Model file for the job. Use its own axes, mm. Round coordinates to 2 decimals unless told otherwise and drop trailing zeros. Loops run counter-clockwise (first coordinate to the right, second up) from the corner with the lowest first, then second, coordinate; pieces in that order, holes last. Notation, with made-up numbers: M 9,3.25 L 60,3.25 A15 ccw 60,20.25 Z; hole C -13.75,-22 d1. An arc over 180 degrees is marked long. Use a Markdown table: item, result. Add a question column.
Q1. Pin check, flat tips, straight feed: pin 1 (7.5 mm diameter, centred on x = -31.75, y = -31.75, fed in from -Z); pin 2 (5 mm diameter, centred on x = -31.75, y = 31.75, fed in from +Z) (3 decimals); pin 3 (8.5 mm diameter, centred on x = 31.75, y = 31.75, fed in from -Z). Stop position of each tip, or through.
Q2. Cut at C-C (y = 0). Give the cut face in (x, z).
Q3. Probe line 1 (Y direction, x = -24, z = -6.25); line 2 (X direction, y = -26.5, z = -10.75); line 3 (Y direction, x = 1, z = -20.25). List the from-to ranges inside material, lowest first. Write a range as from..to.
Q4. Mould opens along Y. For faces 1 (the face through (4.13, 31.48, -9.46)), 2 (the face through (23.289, -23.289, -12.198)), 3 (the face through (1, 50.8, -14)) say: +Y half, -Y half, draft (parallel to the pull), parting line (faces both ways), or undercut.
Q5. Cut at D-D (z = -21.5). Give the cut face in (x, y) (3 decimals).
Q6. Cut at A-A (z = -3.5). Give the cut face in (x, y) (3 decimals).
Q7. Cut at B-B (x = 23). Give the cut face in (y, z), plus the area to 3 significant figures.
from build123d import *

# Parameters (mm, degrees)
F2_DEPTH      = 50.8
F2_DEPTH_BACK = 50.8
F3_D          = 6.35
F5_D          = 63.5


with BuildPart() as f2:
    # F1 (on Right) → F2 (new body, two sides)
    with BuildSketch(Plane.YZ) as f2_sk:
        Polygon((50.8, 0), (-50.8, 0), (-50.8, -6.35), (50.8, -27.945747), align=None)
    extrude(amount=F2_DEPTH)
    extrude(f2_sk.sketch, amount=-F2_DEPTH_BACK)

    # F3 (through all)
    with Locations(Plane.XY):
        with Locations((-31.75, 31.75), (31.75, 31.75), (31.75, -31.75), (-31.75, -31.75)):
            Hole(F3_D / 2)

    # F5 (through all)
    with Locations(Plane.XY):
        with Locations((0, 0)):
            Hole(F5_D / 2)


solid = f2.part
Checked values:
| question | item | result |
|---|---|---|
| 1 | pin 1 | stops at z = -11.2 |
| 1 | pin 2 | passes through |
| 1 | pin 3 | stops at z = -24.8 |
| 2 | outline | M -50.8,-17.15 L -31.75,-17.15 L -31.75,0 L -50.8,0 Z; M 31.75,-17.15 L 50.8,-17.15 L 50.8,0 L 31.75,0 Z |
| 3 | line 1 | y = -50.8..-20.79, 20.79..50.8 |
| 3 | line 2 | x = -50.8..-17.49, 17.49..50.8 |
| 3 | line 3 | y = 31.73..50.8 |
| 4 | face 1 | undercut |
| 4 | face 2 | -Y half |
| 4 | face 3 | +Y half |
| 5 | outline | M -50.8,20.475 L -24.266,20.475 A31.75 cw 24.266,20.475 L 50.8,20.475 L 50.8,50.8 L -50.8,50.8 Z; hole C -31.75,31.75 d6.35; hole C 31.75,31.75 d6.35 |
| 6 | outline | M -50.8,-50.8 L 50.8,-50.8 L 50.8,50.8 L -50.8,50.8 Z; hole C -31.75,-31.75 d6.35; hole C -31.75,31.75 d6.35; hole C 0,0 d63.5; hole C 31.75,-31.75 d6.35; hole C 31.75,31.75 d6.35 |
| 7 | outline | M -50.8,-6.35 L -21.89,-12.5 L -21.89,0 L -50.8,0 Z; M 21.89,-21.8 L 50.8,-27.95 L 50.8,0 L 21.89,0 Z |
| 7 | area | 992 mm^2 |
